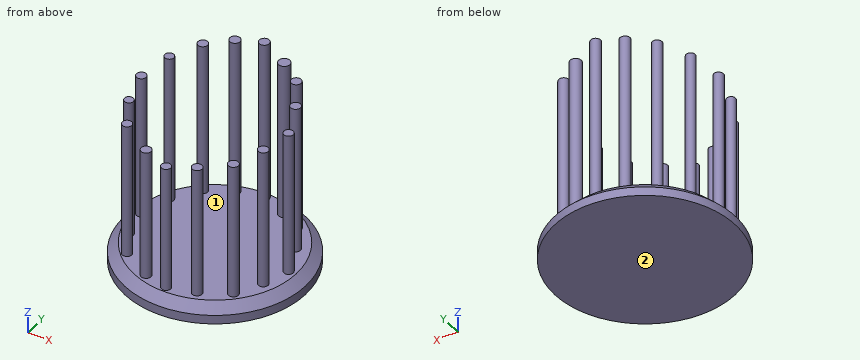
```python
from build123d import *

# Parameters (mm, degrees)
F0_R      = 50
F0_R_2    = 46.581391
F0_R_3    = 2.632067
F0_R_4    = 2.770688
F0_R_5    = 2.478179
F0_R_6    = 2.596253
F0_R_7    = 2.75034
F0_R_8    = 2.770687
F0_R_9    = 2.750345
F0_R_10   = 2.669152
F0_R_11   = 2.523107
F0_R_12   = 2.688372
F0_R_13   = 2.876785
F0_R_14   = 2.605253
F0_R_15   = 2.736693
F0_R_16   = 3.150169
F0_R_17   = 2.750341
F1_DEPTH  = 10
F2_SIZE   = 5.08
F3_DEPTH  = 100
F4_DEPTH  = 97.5
F5_DEPTH  = 95
F6_DEPTH  = 92.5
F7_DEPTH  = 90
F8_DEPTH  = 87.5
F9_DEPTH  = 85
F10_DEPTH = 82.5
F11_DEPTH = 80


with BuildPart() as f1:
    # F0 (on Top) → F1 (new body)
    with BuildSketch(Plane.XY):
        Circle(F0_R)
        Circle(F0_R_2, mode=Mode.SUBTRACT)
        Circle(F0_R_2)
        with Locations((-29.607549, -29.317277)):
            Circle(F0_R_3, mode=Mode.SUBTRACT)
        with Locations((-12.965396, -38.605922)):
            Circle(F0_R_4, mode=Mode.SUBTRACT)
        with Locations((-37.15457, -16.158367)):
            Circle(F0_R_5, mode=Mode.SUBTRACT)
        with Locations((0, -41.508623)):
            Circle(F0_R_6, mode=Mode.SUBTRACT)
        with Locations((14.319992, -37.057813)):
            Circle(F0_R_7, mode=Mode.SUBTRACT)
        with Locations((28.833498, -28.543224)):
            Circle(F0_R_8, mode=Mode.SUBTRACT)
        with Locations((36.187002, -14.416747)):
            Circle(F0_R_9, mode=Mode.SUBTRACT)
        with Locations((-40.831324, 0)):
            Circle(F0_R_10, mode=Mode.SUBTRACT)
        with Locations((-36.380517, 16.93242)):
            Circle(F0_R_11, mode=Mode.SUBTRACT)
        with Locations((-26.89836, 30.865383)):
            Circle(F0_R_12, mode=Mode.SUBTRACT)
        with Locations((-14.126476, 38.605922)):
            Circle(F0_R_13, mode=Mode.SUBTRACT)
        with Locations((40.831324, 0)):
            Circle(F0_R_14, mode=Mode.SUBTRACT)
        with Locations((33.864841, 16.545395)):
            Circle(F0_R_15, mode=Mode.SUBTRACT)
        with Locations((14.707019, 36.283758)):
            Circle(F0_R_16, mode=Mode.SUBTRACT)
        with Locations((0, 41.895645)):
            Circle(F0_R_17, mode=Mode.SUBTRACT)
        with Locations((25.543767, 29.897818)):
            Circle(F0_R_4, mode=Mode.SUBTRACT)
    extrude(amount=F1_DEPTH)

    # F2
    f2_edges = [f1.edges().sort_by_distance(p)[0] for p in [
        (-50, 0, 10),
    ]]
    chamfer(f2_edges, length=F2_SIZE)

    # F0 (on Top) → F3 (join)
    with BuildSketch(Plane.XY):
        with Locations((0, 41.895645)):
            Circle(F0_R_17)
    extrude(amount=F3_DEPTH)

    # F0 (on Top) → F4 (join)
    with BuildSketch(Plane.XY):
        with Locations((-14.126476, 38.605922)):
            Circle(F0_R_13)
        with Locations((14.707019, 36.283758)):
            Circle(F0_R_16)
    extrude(amount=F4_DEPTH)

    # F0 (on Top) → F5 (join)
    with BuildSketch(Plane.XY):
        with Locations((-26.89836, 30.865383)):
            Circle(F0_R_12)
        with Locations((25.543767, 29.897818)):
            Circle(F0_R_4)
    extrude(amount=F5_DEPTH)

    # F0 (on Top) → F6 (join)
    with BuildSketch(Plane.XY):
        with Locations((-36.380517, 16.93242)):
            Circle(F0_R_11)
        with Locations((33.864841, 16.545395)):
            Circle(F0_R_15)
    extrude(amount=F6_DEPTH)

    # F0 (on Top) → F7 (join)
    with BuildSketch(Plane.XY):
        with Locations((40.831324, 0)):
            Circle(F0_R_14)
        with Locations((-40.831324, 0)):
            Circle(F0_R_10)
    extrude(amount=F7_DEPTH)

    # F0 (on Top) → F8 (join)
    with BuildSketch(Plane.XY):
        with Locations((-37.15457, -16.158367)):
            Circle(F0_R_5)
        with Locations((36.187002, -14.416747)):
            Circle(F0_R_9)
    extrude(amount=F8_DEPTH)

    # F0 (on Top) → F9 (join)
    with BuildSketch(Plane.XY):
        with Locations((28.833498, -28.543224)):
            Circle(F0_R_8)
        with Locations((-29.607549, -29.317277)):
            Circle(F0_R_3)
    extrude(amount=F9_DEPTH)

    # F0 (on Top) → F10 (join)
    with BuildSketch(Plane.XY):
        with Locations((14.319992, -37.057813)):
            Circle(F0_R_7)
        with Locations((-12.965396, -38.605922)):
            Circle(F0_R_4)
    extrude(amount=F10_DEPTH)

    # F0 (on Top) → F11 (join)
    with BuildSketch(Plane.XY):
        with Locations((0, -41.508623)):
            Circle(F0_R_6)
    extrude(amount=F11_DEPTH)


solid = f1.part
```
For this review, take the finished solid that the model builds, in its own axes (mm). Face numbers are marked on the shaded views. Give positions to 0.01 mm unless a question says otherwise; leave off trailing zeros. Write each loop counter-clockwise with the first axis right and the second up, starting at its lowest first coordinate (ties: lowest second). Pieces come first, ordered by that corner, then holes. Notation, with made-up numbers: M -5,-15.5 L 53,-15.5 A20 ccw 53,-5.5 Z; hole C 67,-29.75 d1. An arc over 180 degrees is marked long. Answer as a JSON object with one key per item and string values. Group by question number.
Item 1: Draft analysis for pull direction Y (two halves, no side actions). For the marked faces 1 and 2, state which applies: +Y half, -Y half, draft (parallel to the pull), parting line (faces both ways), or undercut.
Item 2: Consider section C-C on x = 0. Write out the cut boundary in (y, z), plus the area to 3 significant figures.
Item 3: For pin 1 Ø8 at (x, z) = (14.5, 50.5) entering from +Y; pin 2 Ø6 at (x, y) = (-26, 31) entering from +Z; pin 3 Ø4 at (y, z) = (28.5, 49.5) entering from +X; pin 4 Ø1.5 at (x, z) = (20, 50) entering from +Y, all flat-tipped, find the tip position at first contact; note any pin that passes through.
Item 4: For probe 1 along Y at (x, z) = (0, 46.5); probe 2 along X at (y, z) = (-39.5, 78); probe 3 along X at (y, z) = (15.5, 33.5), list the stretches that pass through material, from the lowest coordinate up. Write a range as [from, to].
Item 5: Consider section A-A on y = 0. Write out the cut boundary in (x, z), plus the area to 3 significant figures.
Item 6: Consider section B-B on z = 66. Count the separate pieces of the cut face and the enclosed holes in it, plus the area to 3 significant figures.
Check result:
{
 "1": {"face 1": "undercut", "face 2": "draft"},
 "2": {"outline": "M -50,0 L 50,0 L 50,4.92 L 44.92,10 L 44.65,10 L 44.65,100 L 39.15,100 L 39.15,10 L -38.91,10 L -38.91,80 L -44.1,80 L -44.1,10 L -44.92,10 L -50,4.92 Z", "area": "1,830 mm^2"},
 "3": {"pin 1": "stops at y = 39.43", "pin 2": "stops at z = 95", "pin 3": "stops at x = 28.31", "pin 4": "passes through"},
 "4": {"probe 1": "y = [-44.1, -38.91], [39.15, 44.65]", "probe 2": "x = [-15.59, -10.34], [-1.64, 1.64], [13.06, 15.58]", "probe 3": "x = [-38.46, -34.3], [31.34, 36.39]"},
 "5": {"outline": "M -50,0 L 50,0 L 50,4.92 L 44.92,10 L 43.44,10 L 43.44,90 L 38.23,90 L 38.23,10 L -38.16,10 L -38.16,90 L -43.5,90 L -43.5,10 L -44.92,10 L -50,4.92 Z", "area": "1,820 mm^2"},
 "6": {"separate pieces": "16", "enclosed holes": "0", "area": "373 mm^2"}
}
